The drawing under review shows one solid part. Ordinate dimensions are in mm from its lowest x, y, z. Round coordinates to 2 decimals unless told otherwise and drop trailing zeros. Write each loop counter-clockwise with the first axis right and the second up, starting at its lowest first coordinate (ties: lowest second). Pieces come first, ordered by that corner, then holes. Notation, with made-up numbers: (-39, 10.5) -> (-9, 10.5) arc R14 ccw to (-9, 17.5) -> close; hole circle Ø9 at (-12, -36). An arc over 180 degrees is marked (long way). Write item = value, one per line. Start each with the question number.
Item 1: Add section D-D, the plane x = 7.75. State the section outline as (y, z) points, then the cut area to 3 significant figures.
Item 2: For pin 1 Ø6 at (x, z) = (4.5, 10.5) entering from -Y; pin 2 Ø2 at (y, z) = (7.5, 18.5) entering from -X; pin 3 Ø2 at (x, z) = (7.5, 32.5) entering from +Y, all flat-tipped, find the tip position at first contact; note any pin that passes through.
Item 3: Add section C-C, the plane z = 13. State the section outline as (x, y) points.
Item 4: To check wall thickness, follow L1, parallel to X at y = 5.5, z = 25.5; L2, parallel to X at y = 5.25, z = 17; L3, parallel to Y at x = 1.75, z = 3.5. State the ranges of each line that lie inside material, in increasing order.
Item 5: Add section A-A, the plane x = 5. State the section outline as (y, z) points, then the cut area to 3 significant figures.
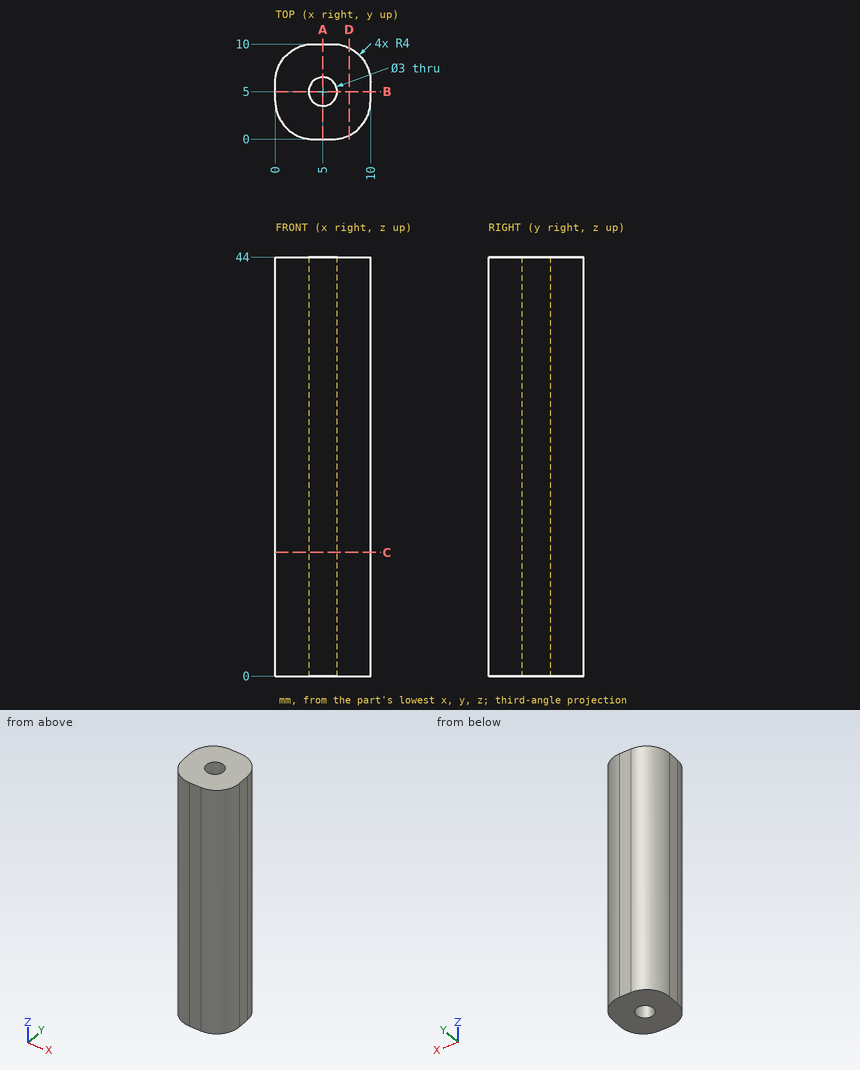
Result set:
q1.outline = (0.4, 0) -> (9.6, 0) -> (9.6, 44) -> (0.4, 44) -> close
q1.area = 405 mm²
q2.pin_1 = 0
q2.pin_2 = 0.03
q2.pin_3 = 9.97
q3.outline = (0, 4) arc R4 ccw to (4, 0) -> (6, 0) arc R4 ccw to (10, 4) -> (10, 6) arc R4 ccw to (6, 10) -> (4, 10) arc R4 ccw to (0, 6) -> close; hole circle Ø3 at (5, 5)
q4.L1 = 0 to 3.59, 6.41 to 10
q4.L2 = 0 to 3.52, 6.48 to 10
q4.L3 = 0.69 to 9.31
q5.outline = (0, 0) -> (3.5, 0) -> (3.5, 44) -> (0, 44) -> close; (6.5, 0) -> (10, 0) -> (10, 44) -> (6.5, 44) -> close
q5.area = 308 mm²
